Could you check a few things on this model? Use its own coordinates, in mm. A direction names the side the tool comes from. Give positions to 0.01 mm unless a question says otherwise; leave off trailing zeros. Write each loop counter-clockwise with the first axis right and the second up, starting at its lowest first coordinate (ties: lowest second). Pieces come first, ordered by that corner, then holes. Notation, with made-up numbers: (3.25, 9.25) - (7.25, 9.25) arc R19 cw to (7.25, 16.25) - close; hole circle Ø9 at (-20, -9). An arc over 180 degrees is marked (long way). Answer in a Markdown table with one row per item.
from build123d import *

# Parameters (mm, degrees)
CROQUIS1_R              = 1.7
SALIENTE_EXTRUIR1_DEPTH = 3


with BuildPart() as part:
    # Croquis1 → Saliente-Extruir1 (new body)
    with BuildSketch(Plane(origin=(0, 0, 0), x_dir=(1, 0, 0), z_dir=(0, 1, 0))):
        with BuildLine():
            Line((-99.377556398, 10.005876847), (-102.377556398, 10.005876847))
            Line((-102.377556398, 10.005876847), (-102.377556398, -73.994123153))
            Line((-102.377556398, -73.994123153), (-99.377556398, -73.994123153))
            Line((-99.377556398, -73.994123153), (-99.377556398, -97.994123153))
            Line((-99.377556398, -97.994123153), (-91.7405656, -96.529736825))
            ThreePointArc((-91.7405656, -96.529736825), (-69.468775837, -90.450126114), (-48.393725101, -81.024813273))
            ThreePointArc((-48.393725101, -81.024813273), (9.137426833, -66.335488141), (66.738359446, -80.748755569))
            ThreePointArc((66.738359446, -80.748755569), (89.168735578, -90.527731735), (112.890583803, -96.529736825))
            Line((112.890583803, -96.529736825), (121.622443602, -97.994123153))
            Line((121.622443602, -97.994123153), (121.622443602, -73.994123153))
            Line((121.622443602, -73.994123153), (124.622443602, -73.994123153))
            Line((124.622443602, -73.994123153), (124.622443602, 10.005876847))
            Line((124.622443602, 10.005876847), (121.622443602, 10.005876847))
            Line((121.622443602, 10.005876847), (121.622443602, 34.005876847))
            Line((121.622443602, 34.005876847), (124.622443602, 34.005876847))
            Line((124.622443602, 34.005876847), (124.622443602, 64.005876847))
            Line((124.622443602, 64.005876847), (121.622443602, 64.005876847))
            Line((121.622443602, 64.005876847), (121.622443602, 89.005112069))
            Line((121.622443602, 89.005112069), (-99.377556398, 89.005839795))
            Line((-99.377556398, 89.005839795), (-99.377556398, 64.005876847))
            Line((-99.377556398, 64.005876847), (-102.377556398, 64.005876847))
            Line((-102.377556398, 64.005876847), (-102.377556398, 34.005876847))
            Line((-102.377556398, 34.005876847), (-99.377556398, 34.005876847))
            Line((-99.377556398, 34.005876847), (-99.377556398, 10.005876847))
        make_face()
        with Locations((-45.378037158, -56.994306397)):
            Circle(CROQUIS1_R, mode=Mode.SUBTRACT)
        with Locations((-45.377872514, -6.994306397)):
            Circle(CROQUIS1_R, mode=Mode.SUBTRACT)
        with Locations((67.622759718, -6.994306397)):
            Circle(CROQUIS1_R, mode=Mode.SUBTRACT)
        with Locations((67.622924362, -56.994306397)):
            Circle(CROQUIS1_R, mode=Mode.SUBTRACT)
    extrude(amount=SALIENTE_EXTRUIR1_DEPTH)


solid = part.part
1) We'd pull the mould along X, two halves only. Please class faces 3 (the face through (10, 3, 3)), 4 (the face through (8.3, 1.48, 66.34)): +X half, -X half, draft (parallel to the pull), parting line (faces both ways), or undercut.
Check values:
| item | result |
|---|---|
| face 3 | draft |
| face 4 | undercut |
2) Imagine slicing it at A-A (z = 85.5). List the corners of the cut face in (x, y) for me.
Check values:
| item | result |
|---|---|
| outline | (-99.38, 0) - (-57.33, 0) - (-57.33, 3) - (-99.38, 3) - close; (76.4, 0) - (121.62, 0) - (121.62, 3) - (76.4, 3) - close |
3) Imagine slicing it at D-D (x = 88.5). List the corners of the cut face in (y, z) for me.
Check values:
| item | result |
|---|---|
| outline | (0, -89.01) - (3, -89.01) - (3, 90.3) - (0, 90.3) - close |
4) Imagine slicing it at C-C (z = -72). List the corners of the cut face in (x, y) for me, then the cut area to 3 significant figures.
Check values:
| item | result |
|---|---|
| outline | (-99.38, 0) - (121.62, 0) - (121.62, 3) - (-99.38, 3) - close |
| area | 663 mm2 |
5) Imagine slicing it at B-B (y = 2.55). List the corners of the cut face in (x, z) for me, then the cut area to 3 significant figures.
Check values:
| item | result |
|---|---|
| outline | (-102.38, -64.01) - (-99.38, -64.01) - (-99.38, -89.01) - (121.62, -89.01) - (121.62, -64.01) - (124.62, -64.01) - (124.62, -34.01) - (121.62, -34.01) - (121.62, -10.01) - (124.62, -10.01) - (124.62, 73.99) - (121.62, 73.99) - (121.62, 97.99) - (112.89, 96.53) arc R150 ccw to (66.74, 80.75) arc R121.14 cw to (-48.39, 81.02) arc R150 ccw to (-91.74, 96.53) - (-99.38, 97.99) - (-99.38, 73.99) - (-102.38, 73.99) - (-102.38, -10.01) - (-99.38, -10.01) - (-99.38, -34.01) - (-102.38, -34.01) - close; hole circle Ø3.4 at (-45.38, 6.99); hole circle Ø3.4 at (-45.38, 56.99); hole circle Ø3.4 at (67.62, 6.99); hole circle Ø3.4 at (67.62, 56.99) |
| area | 38,200 mm2 |
6) Will these pins go through, and if not, where does the flat tip stop? P1, Ø1.5, axis at y = 1.5, z = 88, coming from the -X side; P2, Ø8, axis at x = -63, z = 68.5, coming from the -Y side; P3, Ø1.5, axis at x = -101, y = 2, coming from the -Z side; P4, Ø1.5, axis at x = -101, y = 1, coming from the +Z side.
Check values:
| item | result |
|---|---|
| P1 | stops at x = -99.38 |
| P2 | stops at y = 0 |
| P3 | stops at z = -64.01 |
| P4 | stops at z = 73.99 |
7) If I drill on line 1 (X direction, y = 1.35, z = 6.5); line 2 (Z direction, x = 8, y = 0.2); line 3 (X direction, y = 2.45, z = -76), over which ranges is the centre line in solid material (lowest first)?
Check values:
| item | result |
|---|---|
| line 1 | x = -102.38 to -47, -43.75 to 66, 69.25 to 124.62 |
| line 2 | z = -89.01 to 66.34 |
| line 3 | x = -99.38 to 121.62 |
8) On a 3-axis mill with a long thin cutter (end or side, diameter ignored), from which of +Z, -Z, +X, -X, +Y, -Y can I reach the whole of each face in a straight line? I mean faces 1 (the face through (88.8, 1.5, 90.4)), 2 (the face through (10, 0, 3)). Say none if no direction works.
Check values:
| item | result |
|---|---|
| face 1 | +Z, +Y, -Y |
| face 2 | +Z, -Z, +X, -X, -Y |
